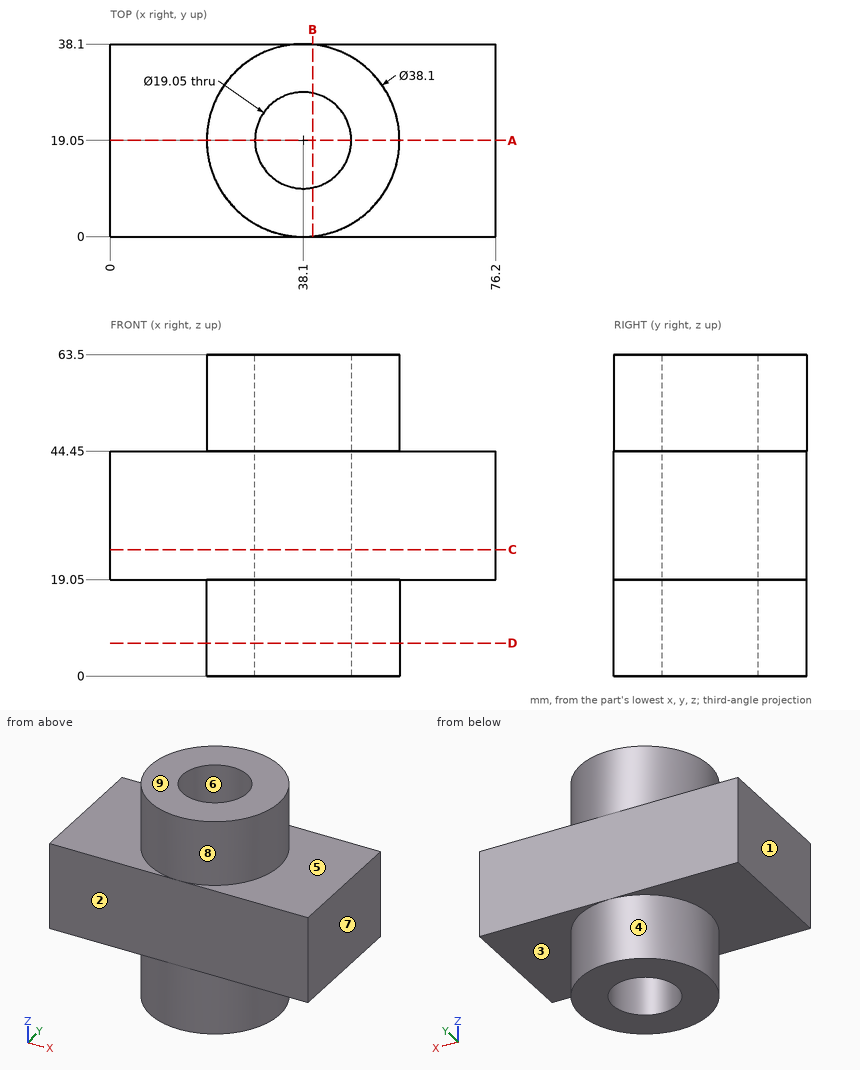
Design review of the part shown in the three views and the two pictorial views. Dimensions are in mm from the part's minimum x, y and z. A direction names the side the tool comes from. Round coordinates to 2 decimals unless told otherwise and drop trailing zeros. Write each loop counter-clockwise with the first axis right and the second up, starting at its lowest first coordinate (ties: lowest second). Pieces come first, ordered by that corner, then holes. Notation, with made-up numbers: (77.5, 66.25) -> (131.5, 66.25) arc R27 ccw to (131.5, 92.25) -> close; hole circle Ø9 at (26, -26). An arc over 180 degrees is marked (long way). Write item = value, one per line. Start each with the question number.
1) Mouldability with a two-part tool opening along X and no side actions: class the marked faces 6, 7, 8 and 9 as +X half, -X half, draft (parallel to the pull), parting line (faces both ways), or undercut.
2) Take a section at C-C, the plane z = 25. State the section outline as (x, y) points (3 decimals), plus the area to 3 significant figures.
3) Take a section at D-D, the plane z = 6.5. State the section outline as (x, y) points (3 decimals), plus the area to 3 significant figures.
4) Take a section at A-A, the plane y = 19.05. State the section outline as (x, z) points (3 decimals), plus the area to 3 significant figures.
5) Wall thickness on probe 1 along Y at (x, z) = (38, 34); probe 2 along X at (y, z) = (19, 49); probe 3 along X at (y, z) = (19, 39): over which ranges is each line inside the solid? List them lowest first. Write a range as from..to.
6) Tool access review of the marked faces 1, 2, 3, 4 and 5: name each direction out of +Z, -Z, +X, -X, +Y, -Y from which nothing blocks a thin tool from reaching the whole face with its end or side.
7) Take a section at B-B, the plane x = 40. State the section outline as (y, z) points, plus the area to 3 significant figures.
8) Clearance check with flat-ended pins moving along their axes: pin 1 (6 mm diameter, centred on y = 16.5, z = 52.5, fed in from -X); pin 2 (6 mm diameter, centred on x = 17.5, y = 5.5, fed in from +Z). State where each tip first meets the part, or that it passes through.
Results list:
q1.face_6 = undercut
q1.face_7 = +X half
q1.face_8 = parting line
q1.face_9 = draft
q2.outline = (0, 0) -> (76.2, 0) -> (76.2, 38.1) -> (0, 38.1) -> close; hole circle Ø19.05 at (38.1, 19.05)
q2.area = 2,620 mm²
q3.outline = circle Ø38.1 at (38.1, 19.05); hole circle Ø19.05 at (38.1, 19.05)
q3.area = 855 mm²
q4.outline = (0, 19.05) -> (19.05, 19.05) -> (19.05, 0) -> (28.575, 0) -> (28.575, 63.5) -> (19.05, 63.5) -> (19.05, 44.45) -> (0, 44.45) -> close; (47.625, 0) -> (57.15, 0) -> (57.15, 19.05) -> (76.2, 19.05) -> (76.2, 44.45) -> (57.15, 44.45) -> (57.15, 63.5) -> (47.625, 63.5) -> close
q4.area = 2,180 mm²
q5.probe_1 = 0..9.53, 28.57..38.1
q5.probe_2 = 19.05..28.58, 47.62..57.15
q5.probe_3 = 0..28.58, 47.62..76.2
q6.face_1 = +Z, -Z, -X, +Y, -Y
q6.face_2 = +Z, -Z, +X, -X, -Y
q6.face_3 = -Z, +X
q6.face_4 = -Z
q6.face_5 = +Z, +X
q7.outline = (0, 19.05) -> (0.09, 19.05) -> (0.09, 0) -> (9.72, 0) -> (9.72, 63.5) -> (0.09, 63.5) -> (0.09, 44.45) -> (0, 44.45) -> close; (28.38, 0) -> (38.01, 0) -> (38.01, 19.05) -> (38.1, 19.05) -> (38.1, 44.45) -> (38.01, 44.45) -> (38.01, 63.5) -> (28.38, 63.5) -> close
q7.area = 1,230 mm²
q8.pin_1 = 19.05
q8.pin_2 = 44.45
